```python
from build123d import *

# Parameters (mm, degrees)
BOSS_EXTRUDE1_DEPTH = 3
SKETCH2_W           = 426
SKETCH2_H           = 199
BOSS_EXTRUDE2_DEPTH = 80
SKETCH3_R           = 5
BOSS_EXTRUDE3_DEPTH = 80


with BuildPart() as part:
    # Sketch1 → Boss-Extrude1 (new body)
    with BuildSketch(Plane.XY):
        Polygon((0, 0), (-24.5, 0), (-24.5, 3), (0, 3), (0, 205), (432, 205), (432, 3), (456.5, 3), (456.5, 0), (432, 0), align=None)
    extrude(amount=BOSS_EXTRUDE1_DEPTH)

    # Sketch2 → Boss-Extrude2 (add)
    with BuildSketch(Plane.XY.offset(3)):
        Polygon((432, 205), (0, 205), (0, 3), (-24.5, 3), (-24.5, 0), (456.5, 0), (456.5, 3), (432, 3), align=None)
        with Locations((216, 102.5)):
            Rectangle(SKETCH2_W, SKETCH2_H, mode=Mode.SUBTRACT)
    extrude(amount=BOSS_EXTRUDE2_DEPTH)

    # Sketch3 → Boss-Extrude3 (add)
    with BuildSketch(Plane.XY.offset(3)):
        with Locations((11, 194)):
            Circle(SKETCH3_R)
        with Locations((421, 194)):
            Circle(SKETCH3_R)
        with Locations((421, 11)):
            Circle(SKETCH3_R)
        with Locations((11, 11)):
            Circle(SKETCH3_R)
    extrude(amount=BOSS_EXTRUDE3_DEPTH)


solid = part.part
```
Work out the finished part from the listing and answer in its coordinate system (mm). A direction names the side the tool comes from. Round coordinates to 2 decimals unless told otherwise and drop trailing zeros. Order: outer loops, then holes, each group sorted by start corner. A loop starts at its lowest first (then second) coordinate and runs counter-clockwise, first axis right, second up.
Q1. A cutting plane is placed at D-D, the plane x = 11. Determine the outline of the cut face in (y, z), then the cut area to 4 significant figures.
Solution:
outline: (0, 0) - (205, 0) - (205, 83) - (202, 83) - (202, 3) - (199, 3) - (199, 83) - (189, 83) - (189, 3) - (16, 3) - (16, 83) - (6, 83) - (6, 3) - (3, 3) - (3, 83) - (0, 83) - close
area: 2,695 mm2
Q2. A tool of negligible diameter and unlimited length cuts with its end or side. For faces 1 (the flat face through (-12, 3, 41)), 2 (the flat face through (219, 104, 3)), 3 (the flat face through (219, 205, 41)), 4 (the flat face through (421, 194, 83)), 5 (the flat face through (432, 103, 41)), from which of +Z, -Z, +X, -X, +Y, -Y can it reach the whole face along a straight path? Write none if from no direction.
Solution:
face 1: +Z, -Z, -X, +Y
face 2: +Z
face 3: +Z, -Z, +X, -X, +Y
face 4: +Z, +X, -X, +Y, -Y
face 5: +Z, -Z, +X, +Y
Q3. The mould has two halves that part along X. Classify faces 6 (the cylindrical face through (425.77, 12.5, 42.44)), 7 (the flat face through (0, 105, 41)), 8 (the flat face through (166, 104, 0)): pulls with the +X half, pulls with the -X half, needs draft (parallel to the pull), parting line crosses it, or undercut.
Solution:
face 6: undercut
face 7: pulls with the -X half
face 8: needs draft
Q4. A cutting plane is placed at C-C, the plane y = 22. Determine the outline of the cut face in (x, z), then the cut area to 3 significant figures.
Solution:
outline: (0, 0) - (432, 0) - (432, 83) - (429, 83) - (429, 3) - (3, 3) - (3, 83) - (0, 83) - close
area: 1,780 mm2
Q5. Find the intervals of material crossed by line 1 along Y through (x, z) = (289, 28.5); line 2 along X through (y, z) = (48, 52); line 3 along Z through (x, y) = (110, 82.5), in increasing order.
Solution:
line 1: y = 0 to 3, 202 to 205
line 2: x = 0 to 3, 429 to 432
line 3: z = 0 to 3
Q6. A cutting plane is placed at B-B, the plane x = 252. Determine the outline of the cut face in (y, z), then the cut area to 4 significant figures.
Solution:
outline: (0, 0) - (205, 0) - (205, 83) - (202, 83) - (202, 3) - (3, 3) - (3, 83) - (0, 83) - close
area: 1,095 mm2
Q7. A cutting plane is placed at A-A, the plane z = 77.5. Determine the outline of the cut face in (x, y).
Solution:
outline: (-24.5, 0) - (456.5, 0) - (456.5, 3) - (432, 3) - (432, 205) - (0, 205) - (0, 3) - (-24.5, 3) - close; circle Ø10 at (11, 11); circle Ø10 at (11, 194); circle Ø10 at (421, 11); circle Ø10 at (421, 194); hole (3, 3) - (429, 3) - (429, 202) - (3, 202) - close
Q8. Given pin 1 Ø12 at (x, z) = (440.5, 60) entering from +Y; pin 2 Ø12 at (y, z) = (84, 46.5) entering from +X; pin 3 Ø4 at (y, z) = (67.5, 14) entering from -X, each flat-ended and moving along its own axis, determine where each tip first touches the part or whether it passes through.
Solution:
pin 1: stops at y = 3
pin 2: stops at x = 432
pin 3: stops at x = 0
